The model under review builds one solid part; all positions refer to its coordinate system, in mm. Face numbers are marked on the shaded views. A direction names the side the tool comes from. Coordinates: 2 decimals unless noted, no trailing zeros. Write each loop counter-clockwise with the first axis right and the second up, starting at its lowest first coordinate (ties: lowest second). Pieces come first, ordered by that corner, then holes. Notation, with made-up numbers: (45, 41) - (50, 41) arc R19 ccw to (50, 76) - close; hole circle Ø11 at (44, 10.5). An arc over 180 degrees is marked (long way). Put each result on its own line as item: value. Start each with the question number.
Item 1: Machinability: for the marked faces 4, 5 and 6, which of the approach directions +Z, -Z, +X, -X, +Y, -Y give a long, thin tool a straight path to every point of the face, cutting with its end or side? Answer none if there is none.
Item 2: Consider section B-B on z = -17.7. Give the boundary of the cut face in (x, y), then the cut area to 3 significant figures.
Item 3: Consider section C-C on x = 3. Give the boundary of the cut face in (y, z), then the cut area to 4 significant figures.
Item 4: Consider section D-D on z = -5.3. Give the boundary of the cut face in (x, y).
Item 5: To check wall thickness, follow L1, parallel to X at y = 0, z = -3.75; L2, parallel to Y at x = 23.8, z = -5.3; L3, parallel to X at y = 7, z = -13. State the ranges of each line that lie inside material, in increasing order. Write a range as [from, to].
Item 6: For pin 1 (1.5 mm diameter, centred on y = -14, z = -20.5, fed in from -X); pin 2 (8 mm diameter, centred on y = 3.5, z = -9.5, fed in from +X); pin 3 (5.5 mm diameter, centred on y = 8, z = -5.3, fed in from +X), all flat-tipped, find the tip position at first contact; note any pin that passes through.
Item 7: Mouldability with a two-part tool opening along Y and no side actions: class the marked faces 1, 2 and 3 as pulls with the +Y half, pulls with the -Y half, needs draft (parallel to the pull), parting line crosses it, or undercut.
Item 8: Consider section A-A on y = 8. Give the boundary of the cut face in (x, z), then the cut area to 3 significant figures.
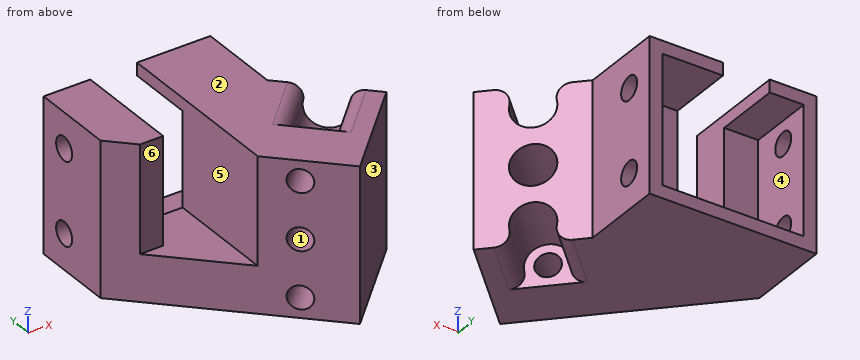
```python
from build123d import *

# Parameters (mm, degrees)
SKETCH1_W           = 25
SKETCH1_H           = 23
BOSS_EXTRUDE1_DEPTH = 12.5
SKETCH4_W           = 21.2
SKETCH4_H           = 19.2
CUT_EXTRUDE2_DEPTH  = 10
BOSS_EXTRUDE2_DEPTH = 23
SKETCH2_W           = 7
SKETCH2_H           = 16
CUT_EXTRUDE1_DEPTH  = 16
BOSS_EXTRUDE3_DEPTH = 23
SKETCH7_R           = 1.75
CUT_EXTRUDE3_DEPTH  = 35.016504294
SKETCH8_R           = 3.05
CUT_EXTRUDE8_DEPTH  = 10
FILLET1_R           = 2
CUT_EXTRUDE9_DEPTH  = 2
SKETCH11_R          = 1.75
CUT_EXTRUDE10_DEPTH = 26
CUT_EXTRUDE11_DEPTH = 14


with BuildPart() as part:
    # Sketch1 → Boss-Extrude1 (new body)
    with BuildSketch(Plane(origin=(0, 0, 0), x_dir=(1, 0, 0), z_dir=(0, 1, 0))):
        with Locations((12.5, 11.5)):
            Rectangle(SKETCH1_W, SKETCH1_H)
    extrude(amount=BOSS_EXTRUDE1_DEPTH)

    # Sketch4 → Cut-Extrude2 (cut)
    with BuildSketch(Plane(origin=(0, 12.5, 0), x_dir=(1, 0, 0), z_dir=(0, 1, 0))):
        with Locations((12.5, 11.5)):
            Rectangle(SKETCH4_W, SKETCH4_H)
    extrude(amount=-CUT_EXTRUDE2_DEPTH, mode=Mode.SUBTRACT)

    # Sketch5 → Boss-Extrude2 (add)
    with BuildSketch(Plane.XY):
        Polygon((25, 0), (12.5, -12.5), (0, 0), align=None)
    extrude(amount=-BOSS_EXTRUDE2_DEPTH)

    # Sketch2 → Cut-Extrude1 (cut)
    with BuildSketch(Plane(origin=(0, 12.5, 0), x_dir=(1, 0, 0), z_dir=(0, 1, 0))):
        with Locations((10.5, 8)):
            Rectangle(SKETCH2_W, SKETCH2_H)
    extrude(amount=-CUT_EXTRUDE1_DEPTH, mode=Mode.SUBTRACT)

    # Sketch6 → Boss-Extrude3 (add)
    with BuildSketch(Plane.XY):
        Polygon((35.606601718, -10.606601718), (25, 0), (12.5, -12.5), (23.106601718, -23.106601718), align=None)
    extrude(amount=-BOSS_EXTRUDE3_DEPTH)

    # Sketch7 → Cut-Extrude3 (cut, through all)
    with BuildSketch(Plane(origin=(12.5, 12.5, 0), x_dir=(0, 0, -1), z_dir=(0.707106781, 0.707106781, 0))):
        with Locations((20, -25.17766953)):
            Circle(SKETCH7_R)
        with Locations((3, -25.17766953)):
            Circle(SKETCH7_R)
        with Locations((11.5, -25.17766953)):
            Circle(SKETCH7_R)
    extrude(amount=-CUT_EXTRUDE3_DEPTH, mode=Mode.SUBTRACT)

    # Sketch8 → Cut-Extrude8 (cut)
    with BuildSketch(Plane(origin=(12.5, 12.5, 0), x_dir=(0, 0, -1), z_dir=(0.707106781, 0.707106781, 0))):
        with Locations((20, -25.17766953)):
            Circle(SKETCH8_R)
        with Locations((11.5, -25.17766953)):
            Circle(SKETCH8_R)
        with Locations((3, -25.17766953)):
            Circle(SKETCH8_R)
    extrude(amount=-CUT_EXTRUDE8_DEPTH, mode=Mode.SUBTRACT)

    # Fillet1
    fillet1_edges = [part.edges().sort_by_distance(p)[0] for p in [
        (26.378858223, -8.449926035, 0),
        (27.156675683, -9.227743494, 0),
        (27.156675683, -9.227743494, -23),
        (26.378858223, -8.449926035, -23),
    ]]
    fillet(fillet1_edges, radius=FILLET1_R)

    # Sketch9 → Cut-Extrude9 (cut)
    with BuildSketch(Plane.XY):
        Polygon((7, -7), (14, -14), (14, -3.5), (7, -3.5), (3.5, -3.5), align=None)
    extrude(amount=-CUT_EXTRUDE9_DEPTH, mode=Mode.SUBTRACT)

    # Sketch11 → Cut-Extrude10 (cut, through all)
    with BuildSketch(Plane(origin=(25, 0, 0), x_dir=(0, 0, -1), z_dir=(1, 0, 0))):
        with Locations((5.3, 8)):
            Circle(SKETCH11_R)
        with Locations((17.7, 8)):
            Circle(SKETCH11_R)
    extrude(amount=-CUT_EXTRUDE10_DEPTH, mode=Mode.SUBTRACT)

    # Sketch12 → Cut-Extrude11 (cut)
    with BuildSketch(Plane.XY.offset(-2)):
        Polygon((3.5, -3.5), (14, -3.5), (14, -14), align=None)
    extrude(amount=-CUT_EXTRUDE11_DEPTH, mode=Mode.SUBTRACT)


solid = part.part
```
Report:
1. face 4: +Y
1. face 5: +Z, +Y, -Y
1. face 6: +Z, -X, -Y
2. outline: (0, 0) - (23.11, -23.11) - (35.61, -10.61) - (31.72, -6.72) - (24.65, -13.79) - (21.82, -10.96) - (28.89, -3.89) - (25, 0) - (25, 6.25) - (23.1, 6.25) - (23.1, 2.5) - (1.9, 2.5) - (1.9, 6.25) - (0, 6.25) - close; (0, 9.75) - (1.9, 9.75) - (1.9, 12.5) - (0, 12.5) - close; (23.1, 9.75) - (25, 9.75) - (25, 12.5) - (23.1, 12.5) - close
2. area: 469 mm²
3. outline: (-3, -23) - (12.5, -23) - (12.5, -21.1) - (2.5, -21.1) - (2.5, -1.9) - (12.5, -1.9) - (12.5, 0) - (-3, 0) - close
3. area: 164.5 mm²
4. outline: (0, 0) - (3.5, -3.5) - (7, -3.5) - (7, 2.5) - (1.9, 2.5) - (1.9, 6.25) - (0, 6.25) - close; (0, 9.75) - (1.9, 9.75) - (1.9, 12.5) - (0, 12.5) - close; (14, -14) - (23.11, -23.11) - (35.61, -10.61) - (31.72, -6.72) - (24.65, -13.79) - (21.82, -10.96) - (28.89, -3.89) - (25, 0) - (25, 6.25) - (23.1, 6.25) - (23.1, 2.5) - (14, 2.5) - close; (23.1, 9.75) - (25, 9.75) - (25, 12.5) - (23.1, 12.5) - close
5. L1: [0, 7], [14, 25]
5. L2: [-22.41, -12.94], [-8.97, 6.25], [9.75, 12.5]
5. L3: [0, 1.9], [23.1, 25]
6. pin 1: x = 13.25
6. pin 2: x = 25.5
6. pin 3: x = 25
7. face 1: undercut
7. face 2: needs draft
7. face 3: pulls with the -Y half
8. outline: (0, -23) - (25, -23) - (25, -19.45) - (23.1, -19.45) - (23.1, -21.1) - (1.9, -21.1) - (1.9, -19.45) - (0, -19.45) - close; (0, -15.95) - (1.9, -15.95) - (1.9, -7.05) - (0, -7.05) - close; (0, -3.55) - (1.9, -3.55) - (1.9, -1.9) - (7, -1.9) - (7, 0) - (0, 0) - close; (14, -1.9) - (23.1, -1.9) - (23.1, -3.55) - (25, -3.55) - (25, 0) - (14, 0) - close; (23.1, -15.95) - (25, -15.95) - (25, -7.05) - (23.1, -7.05) - close
8. area: 128 mm²
